Autodesk Inventor part; units mm, degrees
ref_plane "YZ Plane" through (0, 0, 0) normal (1, 0, 0) x (0, 1, 0)
ref_plane "XZ Plane" through (0, 0, 0) normal (0, 1, 0) x (-1, 0, 0)
ref_plane "XY Plane" through (0, 0, 0) normal (0, 0, 1) x (1, 0, 0)
sketch "스케치1" plane through (0, 0, 0) normal (1, 0, 0) x (0, 1, 0)
  line L0 (12, -9.25) -> (-12, -9.25)
  line L1 (-12, -9.25) -> (-12, 9.25)
  line L2 (-12, 9.25) -> (12, 9.25)
  line L3 (12, 9.25) -> (12, -9.25)
  line L4 (12, -9.25) -> (-12, 9.25) construction
  line L5 (-12, -9.25) -> (12, 9.25) construction
  line L6 (12, 7.75) -> (-10.5, 7.75)
  line L7 (-10.5, 7.75) -> (-10.5, 0.75)
  line L8 (-10.5, 0.75) -> (12, 0.75)
  line L9 (12, 0.75) -> (12, 7.75)
  line L10 (-10.5, -7.75) -> (12, -7.75)
  line L11 (-10.5, -0.75) -> (-10.5, -7.75)
  line L12 (12, -0.75) -> (-10.5, -0.75)
  line L13 (12, 9.25) -> (13.5, 9.25)
  line L14 (13.5, 9.25) -> (13.5, -9.25)
  line L15 (13.5, -9.25) -> (12, -9.25)
  line L16 (12, -9.25) -> (12, 9.25)
  point P0 (0, 0)
  point P1 (12, -7.75)
  point P2 (12, -0.75)
  point P3 (-10, 7.75)
  point P4 (-10, -7.75)
  point P5 (-10, 0.75)
  point P6 (-10, -0.75)
  point P7 (-10, -0.75)
  point P8 (-10, -7.75)
  point P9 (12, 7.75)
  point P10 (12, -7.75)
  dimension "d0" = 24
  dimension "d1" = 18.5
  dimension "d2" = 22.5
  dimension "d3" = 7
  dimension "d4" = 1.5
  dimension "d7" = 8.5
  dimension "d18" = 1.5
extrude "돌출1" add sketch "스케치1" against normal blind 45 contours L0 L1 L2 L3 L6 L7 L8 L12 L11 L10
sketch "스케치2" plane through (0, 0, 0) normal (1, 0, 0) x (0, 0, -1)
  line L0 (-9.25, -12) -> (9.25, -12)
  line L1 (-9.25, 12) -> (-9.25, -12)
  line L2 (-9.25, 12) -> (9.25, 12)
  line L3 (9.25, 12) -> (9.25, -12)
  line L4 (9.25, -12) -> (-9.25, -12)
  line L5 (-9.25, -12) -> (-9.25, 12)
  line L6 (9.25, 12) -> (-9.25, 12)
  line L7 (-9.25, 12) -> (-7.75, 12)
  point P0 (0, 0)
extrude "돌출2" add sketch "스케치2" along normal blind 1
sketch "스케치4" plane through (-45, -12, 9.25) normal (0, 0, 1) x (1, 0, 0)
  circle A0 centre (8.5, 19) radius 1.25
  circle A1 centre (26.5, 19) radius 1.25
  circle A2 centre (26.5, 4) radius 1.25
  circle A3 centre (8.5, 4) radius 1.25
  point P0 (45, 12)
extrude "돌출3" cut sketch "스케치4" against normal blind 45
sketch "스케치9" plane through (0, 12, 7.75) normal (0, 1, 0) x (1, 0, 0)
  line L0 (-45, 7) -> (-45, 8.5)
  line L1 (0, 7) -> (-45, 7)
  line L2 (-45, -1.5) -> (1, -1.5)
  line L3 (-45, 17) -> (1, 17)
  line L4 (-45, 17) -> (-35, 17)
  line L5 (-45, -1.5) -> (-35, -1.5)
  line L6 (-35, -1.5) -> (-35, -11.5)
  line L7 (-35, -11.5) -> (-45, -11.5)
  line L8 (-45, -11.5) -> (-45, -1.5)
  circle A0 centre (-40, -6.5) radius 2
  line L9 (-45, 7.75) -> (0, 7.75) construction
  line L10 (-22, -1.5) -> (-22, 17) construction
  line L11 (-35, 17) -> (-35, 27)
  line L12 (-35, 27) -> (-45, 27)
  line L13 (-45, 27) -> (-45, 17)
  circle A1 centre (-40, 22) radius 2
  line L14 (-45, 17) -> (-35, 17)
  line L15 (1, 17) -> (-9, 17)
  line L16 (1, -1.5) -> (-9, -1.5)
  line L17 (-9, -1.5) -> (-9, -11.5)
  line L18 (-9, -11.5) -> (1, -11.5)
  line L19 (1, -11.5) -> (1, -1.5)
  circle A2 centre (-4, -6.5) radius 2
  circle A3 centre (-4, 22) radius 2
  line L20 (-9, 17) -> (-9, 27)
  line L21 (-9, 27) -> (1, 27)
  line L22 (1, 27) -> (1, 17)
  line L23 (1, 17) -> (-9, 17)
  point P0 (-9, 17)
  dimension "d31" = 10
  dimension "d32" = 10
  dimension "d33" = 4
  dimension "d34" = 5
  dimension "d35" = 5
extrude "돌출6" add sketch "스케치9" against normal blind 1.5
sketch "스케치10" plane through (0, 0, 0) normal (-1, 0, 0) x (0, 0, 1)
  line L0 (-0.75, -10.5) -> (-0.75, 12)
  line L1 (-7.75, 12) -> (-0.75, 12)
  line L2 (-7.75, 12) -> (-7.75, -10.5)
  line L3 (-7.75, -10.5) -> (-0.75, -10.5)
  line L4 (1.75, 9.5) -> (1.75, -10.5)
  line L5 (1.75, -10.5) -> (7.75, -10.5)
  line L6 (7.75, 9.5) -> (7.75, -10.5)
  line L7 (1.75, 9.5) -> (7.75, 9.5)
  line L8 (0.75, 12) -> (0.75, -10.5)
  line L9 (0.75, -10.5) -> (7.75, -10.5)
  line L10 (7.75, -10.5) -> (7.75, 12)
  line L11 (0.75, 12) -> (7.75, 12)
  point P0 (0, 0)
  point P1 (1.75, -10.5)
  point P2 (1.75, 10.75)
  point P3 (7.75, 9.5)
extrude "돌출7" cut sketch "스케치10" against normal blind 10
sketch "스케치11" plane through (-45, -10.5, 7.75) normal (0, 1, 0) x (1, 0, 0)
  line L0 (0, 15.5) -> (46, 15.5)
  line L1 (0, 8.5) -> (0, 15.5)
  line L2 (46, 15.5) -> (46, 8.5)
  line L3 (0, 8.5) -> (0, 7)
  line L4 (46, 8.5) -> (0, 8.5)
  line L5 (46, 8.5) -> (46, 7)
  line L6 (0, 7.75) -> (46, 7.75) construction
  line L7 (23, 15.5) -> (23, 8.5) construction
  line L8 (0, 12) -> (46, 12) construction
  line L9 (4, 9.5) -> (42, 9.5)
  line L10 (42, 9.5) -> (42, 14.5)
  line L11 (42, 14.5) -> (4, 14.5)
  line L12 (4, 14.5) -> (4, 9.5)
  line L13 (4, 9.5) -> (42, 14.5) construction
  line L14 (42, 9.5) -> (4, 14.5) construction
  line L15 (4, 6) -> (42, 6)
  line L16 (42, 6) -> (42, 1)
  line L17 (42, 1) -> (4, 1)
  line L18 (4, 1) -> (4, 6)
  line L19 (0, 7.75) -> (46, 7.75) construction
  line L20 (0, 8.5) -> (46, 8.5)
  point P0 (45, 7.75)
  point P1 (23, 12)
  dimension "d40" = 1
  dimension "d41" = 4
extrude "돌출8" cut sketch "스케치11" against normal blind 10 contours L12 L11 L10 L9 | L15 L16 L17 L18
properties part number "convertor_base" material "고무, 검은색"
CAD build for the part. Positions are in the model's coordinates, mm. A direction names the side the tool comes from. Round coordinates to 2 decimals unless told otherwise and drop trailing zeros. Loops run counter-clockwise (first coordinate to the right, second up) from the corner with the lowest first, then second, coordinate; pieces in that order, holes last. Notation, with made-up numbers: M 57.25,33.25 L 86.25,33.25 A31 cw 86.25,66.25 Z; hole C 22,-29.75 d5. An arc over 180 degrees is marked long. One line per question, with ' | ' between items. Start each with the question number.
Item 1: Cut at B-B, the plane x = -4. State how many separate pieces and enclosed holes the cut face has, plus the area to 3 significant figures.
Item 2: Which spindle directions (+Z, -Z, +X, -X, +Y, -Y) get a long thin tool onto all of the face, cutting with end or side? Do faces 4 (the flat face through (-22, 1, -7.75)), 5 (the flat face through (-22, -11, -6.75)), 6 (the cylindrical face through (-37.49, 6.24, -8.49)), 7 (the flat face through (-37.8, 10.5, 14.2)), 8 (the flat face through (-9, 11, -14)). Say none if no direction does.
Item 3: Cut at A-A, the plane z = 14.25. Write the cut outline in (x, y), plus the area to 3 significant figures.
Item 4: Pin check, flat tips, straight feed: pin 1 Ø1 at (x, y) = (-33.5, 2.5) entering from +Z; pin 2 Ø3 at (x, z) = (-40, 13.5) entering from -Y; pin 3 Ø4 at (x, y) = (-18.5, 7) entering from -Z. Stop position of each tip, or through.
Item 5: Wall check: line 1 (Z direction, x = -4, y = 11.6); line 2 (Z direction, x = -25.5, y = 8); line 3 (Y direction, x = -18.5, z = 0.45). Give the ranges that are in metal, low to high.
Item 6: Two-plate mould, pull along X, no slides. Class faces 1 (the flat face through (-45, 1, 0)), 2 (the flat face through (-41, -11, -4)), 3 (the flat face through (-22, 12, -8)): pulls with the +X half, pulls with the -X half, needs draft (parallel to the pull), parting line crosses it, or undercut.
Item 7: Cut at D-D, the plane y = 9.75. Write the cut outline in (x, z).
Item 8: Cut at C-C, the plane x = -21. Write the cut outline in (y, z), plus the area to 3 significant figures.
Responses:
1) separate pieces: 5 | enclosed holes: 0 | area: 132 mm²
2) face 4: +X, -X, +Y | face 5: +Y, -Y | face 6: +Z, -Z | face 7: +Z, +X, -X, -Y | face 8: -Z, +Y, -Y
3) outline: M -45,10.5 L -42,10.5 L -42,12 L -45,12 Z; M -38,10.5 L -35,10.5 L -35,12 L -38,12 Z; M -9,10.5 L -6,10.5 L -6,12 L -9,12 Z; M -2,10.5 L 1,10.5 L 1,12 L -2,12 Z | area: 18.0 mm²
4) pin 1: stops at z = 9.25 | pin 2: stops at y = 10.5 | pin 3: stops at z = -9.25
5) line 1: z = -19.25 to -16.25, -12.25 to -7.75, -0.75 to 0.75, 7.75 to 12.25, 16.25 to 19.25 | line 2: z = -9.25 to -7.75, -0.75 to 0.75, 7.75 to 9.25 | line 3: y = -12 to -9.25, -6.75 to 5.75, 8.25 to 12
6) face 1: pulls with the -X half | face 2: undercut | face 3: needs draft
7) outline: M -45,-9.25 L 1,-9.25 L 1,-7.75 L -45,-7.75 Z; M -45,-0.75 L 1,-0.75 L 1,0.75 L -45,0.75 Z; M -45,7.75 L 1,7.75 L 1,9.25 L -45,9.25 Z
8) outline: M -12,-9.25 L 12,-9.25 L 12,-7.75 L -10.5,-7.75 L -10.5,-6.75 L -12,-6.75 Z; M -12,-1.75 L -10.5,-1.75 L -10.5,-0.75 L 12,-0.75 L 12,0.75 L -10.5,0.75 L -10.5,1.75 L -12,1.75 Z; M -12,6.75 L -10.5,6.75 L -10.5,7.75 L 12,7.75 L 12,9.25 L -12,9.25 Z | area: 114 mm²
